```python
from build123d import *

# Parameters (mm, degrees)
F0_R     = 95.25
F1_DEPTH = 3.175
F3_DEPTH = 6.35
F4_R     = 6.34999


# Not quite as in the source:
# - a fillet or chamfer is up to 0.001 mm smaller than in the source, because OpenCascade refuses the exact size


with BuildPart() as f1:
    # F0 (on Top) → F1 (new body)
    with BuildSketch(Plane.XY):
        Circle(F0_R)
    extrude(amount=F1_DEPTH)

    # F2 (on Front) → F3 (join, symmetric)
    with BuildSketch(Plane.XZ):
        with BuildLine():
            Line((38.1, 0), (38.1, 25.4))
            Line((38.1, 25.4), (16.9333333333, 44.3320422095))
            ThreePointArc((16.9333333333, 44.3320422095), (0, 50.8), (-16.9333333333, 44.3320422095))
            Line((-16.9333333333, 44.3320422095), (-38.1, 25.4))
            Line((-38.1, 25.4), (-38.1, 0))
            Line((-38.1, 0), (0, 0))
            Line((0, 0), (38.1, 0))
        make_face()
        with BuildLine():
            ThreePointArc((6.35, 38.1), (4.4901280605, 33.6098719395), (0, 31.75))
            ThreePointArc((0, 31.75), (-4.4901280605, 42.5901280605), (6.35, 38.1))
        make_face(mode=Mode.SUBTRACT)
    extrude(amount=F3_DEPTH, both=True)

    # F4 (radius 6.35 in the source; OpenCascade refuses exactly that, so slightly less here)
    f4_edges = [f1.edges().sort_by_distance(p)[0] for p in [
        (-38.1, -6.35, 14.2875),
        (-38.1, 6.35, 14.2875),
        (38.1, -6.35, 14.2875),
        (38.1, 6.35, 14.2875),
    ]]
    fillet(f4_edges, radius=F4_R)


solid = f1.part
```
Could you check a few things on this model? Use its own coordinates, in mm. A direction names the side the tool comes from. Round coordinates to 2 decimals unless told otherwise and drop trailing zeros. Order: outer loops, then holes, each group sorted by start corner. A loop starts at its lowest first (then second) coordinate and runs counter-clockwise, first axis right, second up. Notation, with made-up numbers: (27, -39) -> (85, -39) arc R24 ccw to (85, -24) -> close; hole circle Ø9 at (-8.5, 30.25). An arc over 180 degrees is marked (long way). One line per question, with ' | ' between items.
Q1. If we section it at A-A on x = 0: Write out the boundary of the cut face in (y, z) (3 decimals).
Computed values:
outline: (-95.25, 0) -> (95.25, 0) -> (95.25, 3.175) -> (6.35, 3.175) -> (6.35, 31.75) -> (-6.35, 31.75) -> (-6.35, 3.175) -> (-95.25, 3.175) -> close; (-6.35, 44.45) -> (6.35, 44.45) -> (6.35, 50.8) -> (-6.35, 50.8) -> close
Q2. Which directions (+Z, -Z, +X, -X, +Y, -Y) give clear straight access to the entire face, cutting with the end or side of a thin tool? Please do faces 5 (the face through (0, -6.35, 22)), 6 (the face through (-36.19, 4.54, 13.83)), 7 (the face through (0, 6.35, 22)), 8 (the face through (-36.29, -4.44, 13.83)), 9 (the face through (36.29, 4.44, 14.22)).
Computed values:
face 5: +Z, +X, -X, -Y | face 6: +Z, -X, +Y | face 7: +Z, +X, -X, +Y | face 8: +Z, -X, -Y | face 9: +Z, +X, +Y
Q3. If I drill on line 1 (Z direction, x = 0, y = -1); line 2 (Z direction, x = 7, y = 57.5) (3 decimals); line 3 (X direction, y = -0.75, z = 38.1), over which ranges is the centre line in solid material (lowest first)? Write a range as from..to.
Computed values:
line 1: 0..31.75, 44.45..50.8 | line 2: 0..3.175 | line 3: -23.9..-6.35, 6.35..23.9
Q4. We'd pull the mould along X, two halves only. Please class faces 1 (the face through (-75.587, -57.958, 1.565)), 2 (the face through (27.7, -0.1, 34.7)), 3 (the face through (-1, -1, 0)), 4 (the face through (-6.344, 0.089, 37.821)): released by +X, released by -X, zero draft, split by the parting line, or undercut.
Computed values:
face 1: split by the parting line | face 2: released by +X | face 3: zero draft | face 4: undercut
Q5. If we section it at B-B on z = 38.1: Write out the boundary of the cut face in (x, y), plus the area to 3 significant figures.
Computed values:
outline: (-23.9, -6.35) -> (-6.35, -6.35) -> (-6.35, 6.35) -> (-23.9, 6.35) -> close; (6.35, -6.35) -> (23.9, -6.35) -> (23.9, 6.35) -> (6.35, 6.35) -> close | area: 446 mm²
Q6. I'm going to push flat-ended pins straight in: pin 1 (2 mm diameter, centred on x = 13.5, z = 40, fed in from -Y); pin 2 (14.5 mm diameter, centred on x = -7, z = 18, fed in from +Y); pin 3 (7.5 mm diameter, centred on x = 0, z = 38.1, fed in from -Y); pin 4 (10 mm diameter, centred on x = 5.5, z = 43.5, fed in from -Y). Where does each tip first touch, or does it pass through?
Computed values:
pin 1: y = -6.35 | pin 2: y = 6.35 | pin 3: through | pin 4: y = -6.35
Q7. If we section it at C-C on y = -3: Write out the boundary of the cut face in (x, z) (3 decimals), plus the area to 3 significant figures.
Computed values:
outline: (-95.203, 0) -> (95.203, 0) -> (95.203, 3.175) -> (37.347, 3.175) -> (37.347, 26.074) -> (16.933, 44.332) arc R25.4 ccw to (-16.933, 44.332) -> (-37.347, 26.074) -> (-37.347, 3.175) -> (-95.203, 3.175) -> close; hole circle Ø12.7 at (0, 38.1) | area: 3,330 mm²
Q8. If we section it at D-D on y = 50: Write out the boundary of the cut face in (x, z) (3 decimals), plus the area to 3 significant figures.
Computed values:
outline: (-81.071, 0) -> (81.071, 0) -> (81.071, 3.175) -> (-81.071, 3.175) -> close | area: 515 mm²
